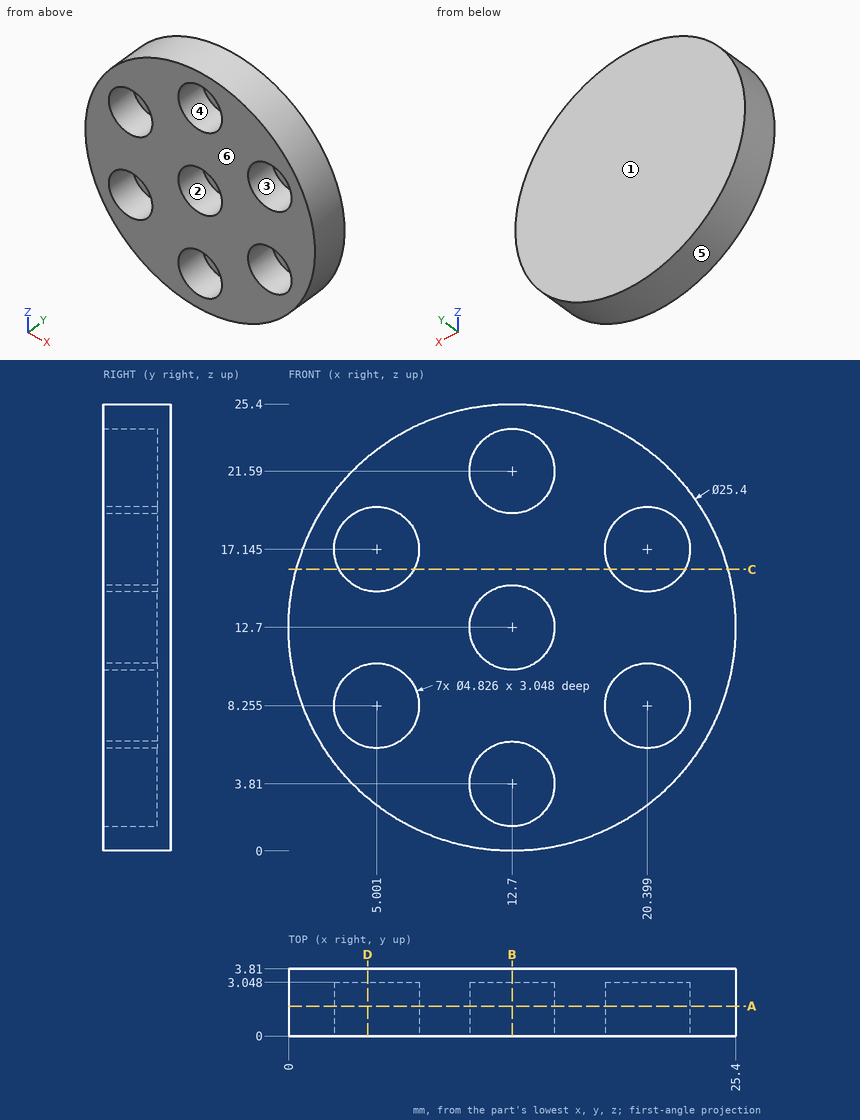
For this review, use the dimensioned drawing (mm, ordinates from the lowest corner) and the shaded views. A direction names the side the tool comes from. Coordinates: 2 decimals unless noted, no trailing zeros. Loops run counter-clockwise (first coordinate to the right, second up) from the corner with the lowest first, then second, coordinate; pieces in that order, holes last.
1. Add section C-C, the plane z = 16. Give the boundary of the cut face in (x, y) (3 decimals).
2. Add section B-B, the plane x = 12.7. Give the boundary of the cut face in (y, z).
3. Add section A-A, the plane y = 1.7. Give the boundary of the cut face in (x, z) (1 decimal), then the cut area to 3 significant figures.
4. For line 1 (Z direction, x = 21, y = 0.95); line 2 (Z direction, x = 6, y = 2.25); line 3 (Z direction, x = 13, y = 2.8), list the stretches that pass through material, from the lowest coordinate up.
5. Insertion check: P1, Ø1.5, axis at x = 20, y = 3, coming from the +Z side; P2, Ø2.5, axis at x = 5, z = 8, coming from the -Y side; P3, Ø1, axis at y = 2, z = 21.5, coming from the +X side. Each pin has a flat end and moves straight along its axis. Give the tip position at first contact, or say it passes through.
6. For the marked faces 1 and 2, list the 3-axis set-ups (+Z, -Z, +X, -X, +Y, -Y) from which the entire face can be reached by the end or side of a thin tool; tool diameter is ignored.
7. Mouldability with a two-part tool opening along Z and no side actions: class the marked faces 3, 4, 5 and 6 as +Z half, -Z half, draft (parallel to the pull), parting line (faces both ways), or undercut.
8. Add section D-D, the plane x = 4.5. Give the boundary of the cut face in (y, z).
Result:
1. outline: (0.436, 0) - (2.877, 0) - (2.877, 3.048) - (7.125, 3.048) - (7.125, 0) - (18.275, 0) - (18.275, 3.048) - (22.523, 3.048) - (22.523, 0) - (24.964, 0) - (24.964, 3.81) - (0.436, 3.81) - close
2. outline: (0, 0) - (3.81, 0) - (3.81, 25.4) - (0, 25.4) - (0, 24) - (3.05, 24) - (3.05, 19.18) - (0, 19.18) - (0, 15.11) - (3.05, 15.11) - (3.05, 10.29) - (0, 10.29) - (0, 6.22) - (3.05, 6.22) - (3.05, 1.4) - (0, 1.4) - close
3. outline: circle Ø25.4 at (12.7, 12.7); hole circle Ø4.8 at (5, 8.3); hole circle Ø4.8 at (5, 17.1); hole circle Ø4.8 at (12.7, 3.8); hole circle Ø4.8 at (12.7, 12.7); hole circle Ø4.8 at (12.7, 21.6); hole circle Ø4.8 at (20.4, 8.3); hole circle Ø4.8 at (20.4, 17.1)
3. area: 379 mm2
4. line 1: z = 3.09 to 5.92, 10.59 to 14.81, 19.48 to 22.31
4. line 2: z = 1.91 to 6.06, 10.45 to 14.95, 19.34 to 23.49
4. line 3: z = 0 to 1.42, 6.2 to 10.31, 15.09 to 19.2, 23.98 to 25.4
5. P1: stops at z = 23.58
5. P2: stops at y = 3.05
5. P3: stops at x = 22.31
6. face 1: +Z, -Z, +X, -X, +Y
6. face 2: -Y
7. face 3: undercut
7. face 4: undercut
7. face 5: parting line
7. face 6: draft
8. outline: (0, 3) - (3.81, 3) - (3.81, 22.4) - (0, 22.4) - (0, 19.51) - (3.05, 19.51) - (3.05, 14.78) - (0, 14.78) - (0, 10.62) - (3.05, 10.62) - (3.05, 5.89) - (0, 5.89) - close
